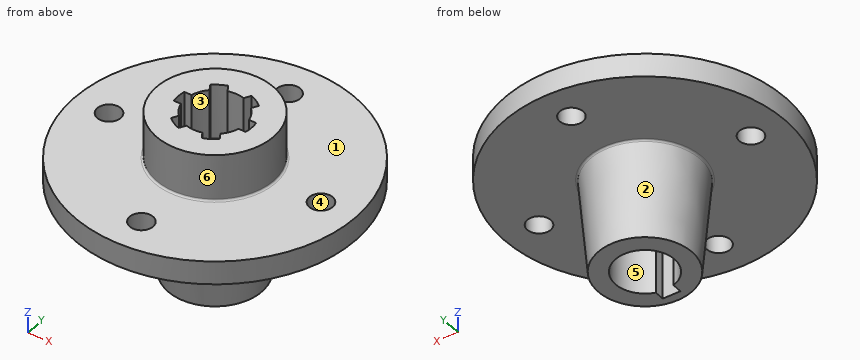
Autodesk Inventor part; units mm, degrees
ref_plane "YZ Plane" through (0, 0, 0) normal (1, 0, 0) x (0, 1, 0)
ref_plane "XZ Plane" through (0, 0, 0) normal (0, 1, 0) x (-1, 0, 0)
ref_plane "XY Plane" through (0, 0, 0) normal (0, 0, 1) x (1, 0, 0)
sketch "Sketch1" plane through (0, 0, 0) normal (0, 0, 1) x (1, 0, 0)
  circle A0 centre (0, 0) radius 38.1
  dimension "d2" = 76.2
extrude "Extrusion1" add sketch "Sketch1" along normal mid plane 6.35
sketch "Sketch2" plane through (0, 0, 3.175) normal (0, 0, 1) x (1, 0, 0)
  circle A0 centre (0, 0) radius 38.1
  point P0 (0, 28.575)
  dimension "d3" = 0
  dimension "d4" = 28.575
hole "Mounting Hole" at (0, 28.575, 3.175) direction (0, 0, -1) diameter 6.35 end through all
pattern_circular "Circular Pattern1" count 4 over 360 about axis through (0, 0, 0) along (0, 0, 1) of "Mounting Hole"
sketch "Sketch3" plane through (0, 0, 3.175) normal (0, 0, 1) x (1, 0, 0)
  circle A0 centre (0, 0) radius 38.1
  circle A1 centre (0, 0) radius 15.875
  dimension "d15" = 31.75
extrude "Extrusion2" add sketch "Sketch3" along normal blind 12.7 contours A1
sketch "Sketch8" plane through (0, 0, 15.875) normal (0, 0, 1) x (1, 0, 0)
  circle A0 centre (0, 0) radius 15.875
hole "Hole3" at (0, 0, 15.875) direction (0, 0, -1) diameter 16.2 depth 14.986
sketch "Sketch4" plane through (0, 0, 15.875) normal (0, 0, 1) x (1, 0, 0)
  arc A0 (-3.0359, 9.528) -> (-6.5275, 7.5757) centre (0, 0) ccw
  circle A1 centre (0, 0) radius 15.875
  line L0 (0, 0) -> (-5, 8.6603) construction
  line L1 (0, 0) -> (-10.16, 0) construction
  line L2 (-2.058, 7.8342) -> (-3.0359, 9.528)
  line L3 (-5.5564, 5.8937) -> (-6.5275, 7.5757)
  arc A2 (-2.058, 7.8342) -> (-5.5564, 5.8937) centre (0, 0) ccw
  circle A3 centre (0, 0) radius 8.1
  dimension "d46" = 60
  dimension "d47" = 4
  dimension "d48" = 20
extrude "Extrusion3" cut sketch "Sketch4" against normal up to surface (14.986 mm away) contours L2 A2 L3 A0
pattern_circular "Circular Pattern2" count 6 over 360 about axis through (0, 0, 0) along (0, 0, 1) of "Extrusion3"
sketch "Sketch5" plane through (0, 0, -3.175) normal (0, 0, -1) x (-1, 0, 0)
  circle A0 centre (0, 0) radius 38.1
  circle A1 centre (0, 0) radius 14.9225
  dimension "d27" = 29.845
extrude "Extrusion4" add sketch "Sketch5" along normal blind 25.4 draft -5 contours A1
sketch "Sketch6" plane through (0, 0, -28.575) normal (0, 0, -1) x (-1, 0, 0)
  circle A0 centre (0, 0) radius 12.7003
  arc A1 (2.3812, -7.6374) -> (-2.3813, -7.6374) centre (0, 0) ccw
  line L0 (-2.3813, -7.6374) -> (-2.3812, -10.3188)
  line L1 (-2.3812, -10.3188) -> (2.3813, -10.3188)
  line L2 (2.3813, -10.3188) -> (2.3812, -7.6374)
  dimension "d31" = 16
  dimension "d32" = 4.7625
  dimension "d33" = 10.3187
extrude "Extrusion5" cut sketch "Sketch6" against normal blind 28.575 contours L2 L1 L0 A1
sketch "Sketch7" plane through (0, 0, 0) normal (0, 0, -1) x (-1, 0, 0)
  arc A0 (2.3812, -7.6374) -> (-2.3813, -7.6374) centre (0, 0) ccw
  point P0 (0, 0)
hole "Hole2" at (0, 0, 0) direction (0, 0, 1) diameter 9.525 end through all
fillet "Fillet1" radius 0.508 2 edges at (14.9225, 0, -3.175) (-15.875, 0, 3.175)
properties part number "Nippon-Denso Gear Coupler" material "ABS Plastic"
Could you check a few things on this model? Use its own coordinates, in mm. Face numbers are marked on the shaded views. A direction names the side the tool comes from. Give positions to 0.01 mm unless a question says otherwise; leave off trailing zeros. Order: outer loops, then holes, each group sorted by start corner. A loop starts at its lowest first (then second) coordinate and runs counter-clockwise, first axis right, second up.
Item 1: If we section it at A-A, the plane z = -12.5: Write out the boundary of the cut face in (x, y), plus the area to 3 significant figures.
Item 2: For the marked faces 4, 5 and 6, which set-ups out of +Z, -Z, +X, -X, +Y, -Y let a thin tool reach every point of the face, with its end or its side?
Item 3: I'm going to push flat-ended pins straight in: pin 1 (3 mm diameter, centred on y = -9, z = -8.5, fed in from +X); pin 2 (5 mm diameter, centred on x = 4, z = -14.5, fed in from +Y); pin 3 (5 mm diameter, centred on y = 1, z = -7, fed in from -X); pin 4 (18.5 mm diameter, centred on x = 0, y = 0, fed in from +Z) (3 decimals). Where does each tip first touch, or does it pass through?
Item 4: If we section it at D-D, the plane z = -18: Write out the boundary of the cut face in (x, y), plus the area to 3 significant figures.
Item 5: If we mould it in two halves opening along X, with no side actions, what happens to the marked faces 1, 2 and 3? For each: pulls with the +X half, pulls with the -X half, needs draft (parallel to the pull), parting line crosses it, or undercut.
Item 6: I need wall thicknesses on line 1 (X direction, y = 9, z = 7.5); line 2 (X direction, y = -1, z = 3); line 3 (Z direction, x = -33.5, y = 16) (3 decimals). Which ranges of each line are inside material? Lowest first, please.
Item 7: If we section it at B-B, the plane x = 0: Count the separate pieces of the cut face and the enclosed holes in it, plus the area to 3 significant figures.
Values:
1. outline: circle Ø28.21 at (0, 0); hole (-2.38, -10.32) - (2.38, -10.32) - (2.38, -7.64) arc R8 ccw (long way) to (-2.38, -7.64) - close
1. area: 412 mm2
2. face 4: +Z, -Z
2. face 5: -Z
2. face 6: +Z
3. pin 1: stops at x = 12.37
3. pin 2: stops at y = 13.92
3. pin 3: stops at x = -14.79
3. pin 4: stops at z = 15.875
4. outline: circle Ø27.25 at (0, 0); hole (-2.38, -10.32) - (2.38, -10.32) - (2.38, -7.64) arc R8 ccw (long way) to (-2.38, -7.64) - close
4. area: 371 mm2
5. face 1: needs draft
5. face 2: parting line crosses it
5. face 3: undercut
6. line 1: x = -13.08 to -4.36, -2.73 to 3.04, 4.36 to 13.08
6. line 2: x = -38.09 to -31.59, -25.56 to -9.95, 9.95 to 25.56, 31.59 to 38.09
6. line 3: z = -3.175 to 3.175
7. separate pieces: 4
7. enclosed holes: 0
7. area: 734 mm2
